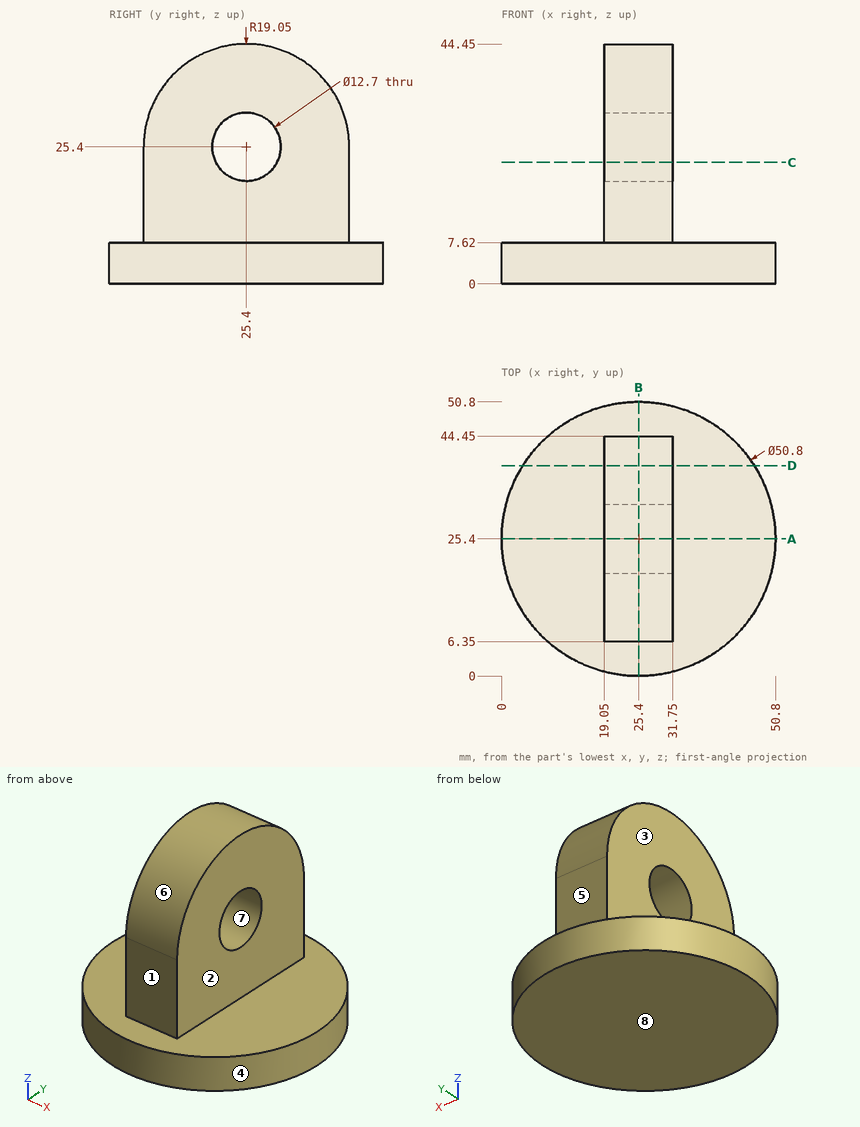
For this review, use the dimensioned drawing (mm, ordinates from the lowest corner) and the shaded views. A direction names the side the tool comes from. Give positions to 0.01 mm unless a question says otherwise; leave off trailing zeros. Write each loop counter-clockwise with the first axis right and the second up, starting at its lowest first coordinate (ties: lowest second). Pieces come first, ordered by that corner, then holes.
(1) Consider section B-B, the plane x = 25.4. Give the boundary of the cut face in (y, z).
(2) Consider section A-A, the plane y = 25.4. Give the boundary of the cut face in (x, z), and give its area (3 significant figures).
(3) Consider section D-D, the plane y = 39. Give the boundary of the cut face in (x, z), and give its area (3 significant figures).
(4) For P1, Ø4, axis at x = 32, z = 27.5, coming from the -Y side; P2, Ø5, axis at x = 19, z = 39, coming from the -Y side; P3, Ø7.5, axis at y = 25.4, z = 25.4, coming from the +X side; P4, Ø12, axis at x = 22, z = 37.5, coming from the +Y side, all flat-tipped, find the tip position at first contact; note any pin that passes through.
(5) Consider section C-C, the plane z = 22.5. Give the boundary of the cut face in (x, y).
(6) The part is to be moulded in two halves that separate along Z. For the marked faces 5, 6, 7 and 8, say which applies: released by +Z, released by -Z, zero draft, split by the parting line, or undercut.
(7) Tool access review of the marked faces 1, 2, 3 and 4: name each direction out of +Z, -Z, +X, -X, +Y, -Y from which nothing blocks a thin tool from reaching the whole face with its end or side.
(8) To check wall thickness, follow L1, parallel to Y at x = 25.75, z = 25.4; L2, parallel to Z at x = 22, y = 25.4; L3, parallel to Z at x = 39.5, y = 37.5. State the ranges of each line that lie inside material, in increasing order.
Returned:
1. outline: (0, 0) - (50.8, 0) - (50.8, 7.62) - (44.45, 7.62) - (44.45, 25.4) arc R19.05 ccw to (6.35, 25.4) - (6.35, 7.62) - (0, 7.62) - close; hole circle Ø12.7 at (25.4, 25.4)
2. outline: (0, 0) - (50.8, 0) - (50.8, 7.62) - (31.75, 7.62) - (31.75, 19.05) - (19.05, 19.05) - (19.05, 7.62) - (0, 7.62) - close; (19.05, 31.75) - (31.75, 31.75) - (31.75, 44.45) - (19.05, 44.45) - close
2. area: 694 mm2
3. outline: (3.95, 0) - (46.85, 0) - (46.85, 7.62) - (31.75, 7.62) - (31.75, 38.74) - (19.05, 38.74) - (19.05, 7.62) - (3.95, 7.62) - close
3. area: 722 mm2
4. P1: stops at y = 6.35
4. P2: stops at y = 9.92
4. P3: passes through
4. P4: stops at y = 43.45
5. outline: (19.05, 6.35) - (31.75, 6.35) - (31.75, 19.75) - (19.05, 19.75) - close; (19.05, 31.05) - (31.75, 31.05) - (31.75, 44.45) - (19.05, 44.45) - close
6. face 5: zero draft
6. face 6: released by +Z
6. face 7: undercut
6. face 8: released by -Z
7. face 1: +Z, +X, -X, -Y
7. face 2: +Z, +X, +Y, -Y
7. face 3: +Z, -X, +Y, -Y
7. face 4: +Z, -Z
8. L1: y = 6.35 to 19.05, 31.75 to 44.45
8. L2: z = 0 to 19.05, 31.75 to 44.45
8. L3: z = 0 to 7.62
